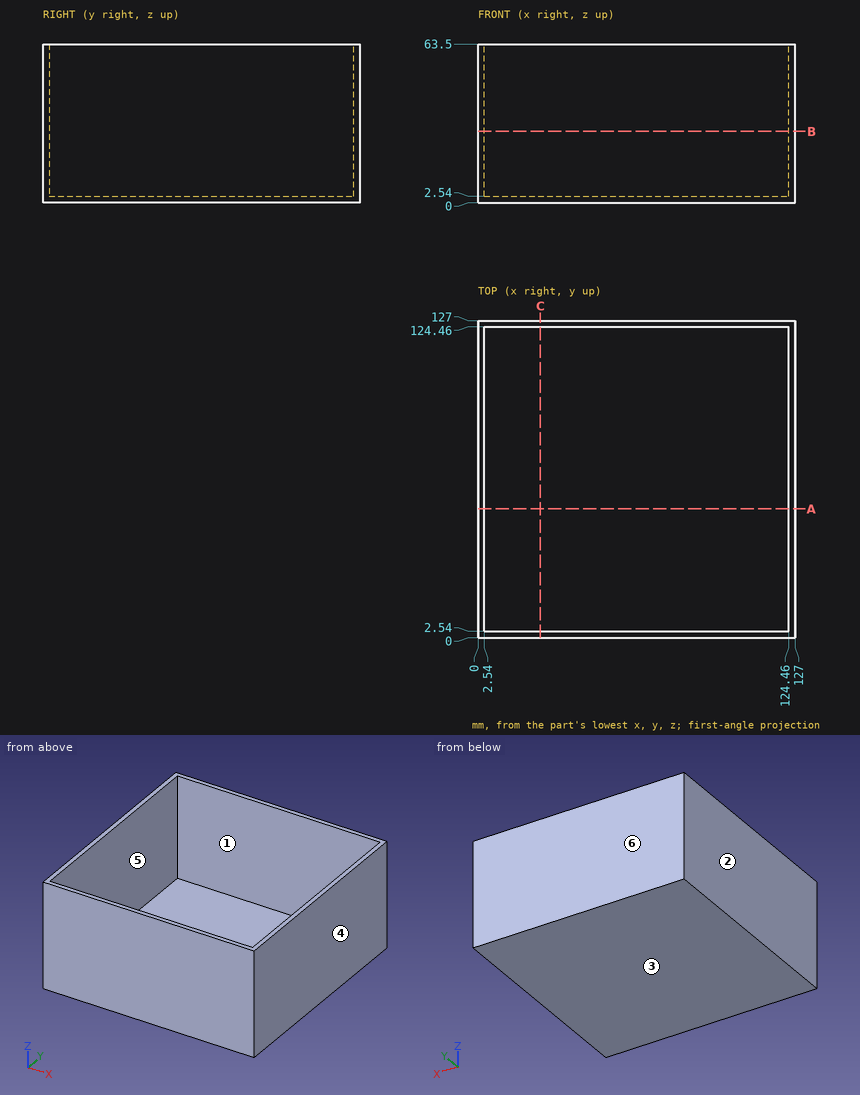
Geometry check sheet. Reference: drawing and pictorial views, mm from the part's lowest x, y, z. A direction names the side the tool comes from. Coordinates: 2 decimals unless noted, no trailing zeros. Loops run counter-clockwise (first coordinate to the right, second up) from the corner with the lowest first, then second, coordinate; pieces in that order, holes last. Notation, with made-up numbers: (25.5, 77) -> (31.5, 77) arc R23 cw to (31.5, 110) -> close; hole circle Ø6 at (69.25, 61). An arc over 180 degrees is marked (long way). Write item = value, one per line. Start each with the question number.
1. Section check B-B on z = 28.5. Record the cut outline in (x, y), then the cut area to 3 significant figures.
2. Material ranges on line 1 (X direction, y = 61, z = 11.5); line 2 (Z direction, x = 94, y = 62.5), recorded low to high.
3. Draft check along X on the marked faces 1, 2, 3 and 4. Enter one of: released by +X, released by -X, zero draft, split by the parting line, or undercut.
4. Depth check by flat-ended pin: P1, Ø5, axis at x = 25, y = 71, coming from the +Z side. Enter the tip coordinate at first touch or a pass-through.
5. Tool access check on the marked faces 5 and 6. Record the directions out of +Z, -Z, +X, -X, +Y, -Y that give a thin tool (end or side, any length) a straight path to the whole face; none if there is none.
6. Section check A-A on y = 51.5. Record the cut outline in (x, z).
Responses:
q1.outline = (0, 0) -> (127, 0) -> (127, 127) -> (0, 127) -> close; hole (2.54, 2.54) -> (124.46, 2.54) -> (124.46, 124.46) -> (2.54, 124.46) -> close
q1.area = 1,260 mm2
q2.line_1 = 0 to 2.54, 124.46 to 127
q2.line_2 = 0 to 2.54
q3.face_1 = undercut
q3.face_2 = released by -X
q3.face_3 = zero draft
q3.face_4 = released by +X
q4.P1 = 2.54
q5.face_5 = +Z
q5.face_6 = +Z, -Z, +X, -X, +Y
q6.outline = (0, 0) -> (127, 0) -> (127, 63.5) -> (124.46, 63.5) -> (124.46, 2.54) -> (2.54, 2.54) -> (2.54, 63.5) -> (0, 63.5) -> close
